Part print with two shaded views. Sizes in mm from the minimum x, y, z corner. A direction names the side the tool comes from. Give positions to 0.01 mm unless a question says otherwise; leave off trailing zeros. Order: outer loops, then holes, each group sorted by start corner. A loop starts at its lowest first (then second) coordinate and runs counter-clockwise, first axis right, second up. Notation, with made-up numbers: M 59.5,55.25 L 90.5,55.25 A29 cw 90.5,78.25 Z; hole C -12,88 d1. An arc over 180 degrees is marked long. Return JSON: item names as keys, results as strings.
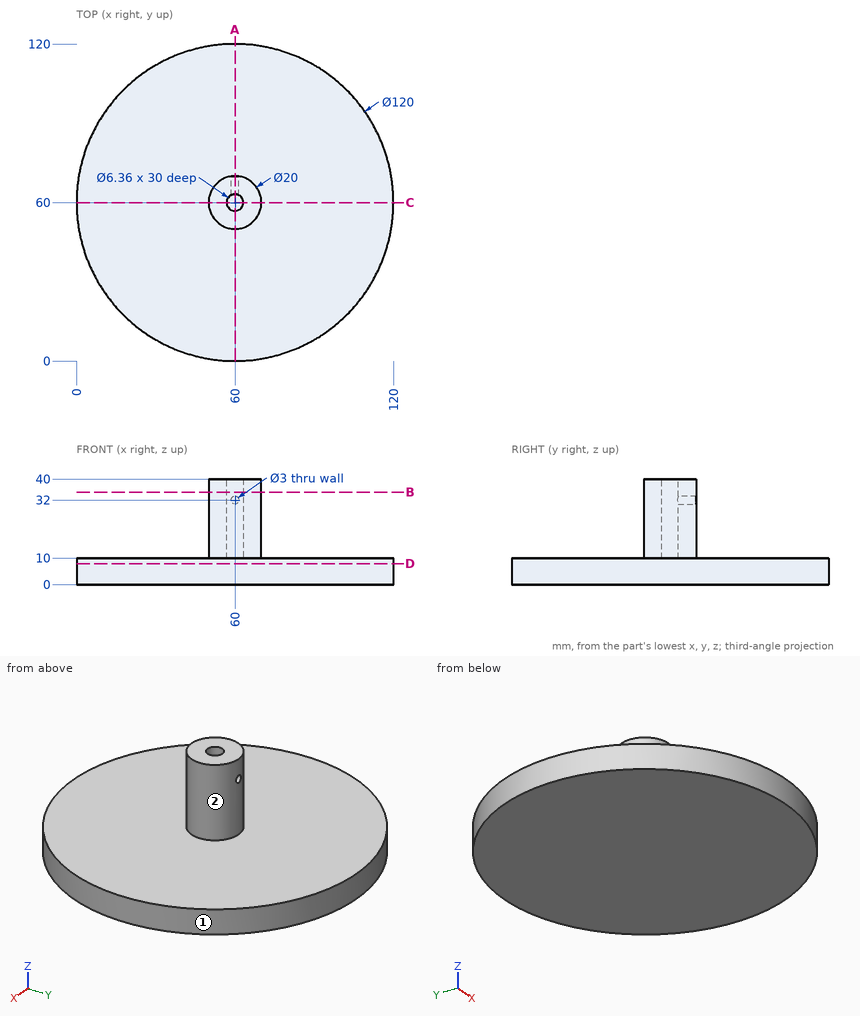
Q1. Band-saw the part on B-B (z = 35). Give the cut face in (x, y).
Established:
{"outline": "C 60,60 d20; hole C 60,60 d6.36"}
Q2. Band-saw the part on C-C (y = 60). Give the cut face in (x, z), then the cut area to 3 significant figures.
Established:
{"outline": "M 0,0 L 120,0 L 120,10 L 70,10 L 70,40 L 63.18,40 L 63.18,10 L 56.82,10 L 56.82,40 L 50,40 L 50,10 L 0,10 Z", "area": "1,610 mm²"}
Q3. Probe line 1 along Y through (x, z) = (60, 17.5); line 2 along Z through (x, y) = (18, 70); line 3 along X through (y, z) = (68, 32). List the from-to ranges inside material, lowest first.
Established:
{"line 1": "y = 50 to 56.82, 63.18 to 70", "line 2": "z = 0 to 10", "line 3": "x = 54 to 58.5, 61.5 to 66"}
Q4. Band-saw the part on A-A (x = 60). Give the cut face in (y, z).
Established:
{"outline": "M 0,0 L 120,0 L 120,10 L 70,10 L 70,30.5 L 63.18,30.5 L 63.18,10 L 56.82,10 L 56.82,40 L 50,40 L 50,10 L 0,10 Z; M 63.18,33.5 L 70,33.5 L 70,40 L 63.18,40 Z"}
Q5. Pin check, flat tips, straight feed: pin 1 (8 mm diameter, centred on x = 97, y = 69.5, fed in from +Z); pin 2 (5 mm diameter, centred on x = 60, z = 32, fed in from -Y); pin 3 (1.5 mm diameter, centred on x = 45.5, z = 4.5, fed in from -Y). Stop position of each tip, or through.
Established:
{"pin 1": "stops at z = 10", "pin 2": "stops at y = 50", "pin 3": "stops at y = 1.6"}
Q6. Band-saw the part on D-D (z = 8). Give the cut face in (x, y), then the cut area to 3 significant figures.
Established:
{"outline": "C 60,60 d120", "area": "11,300 mm²"}
Q7. 3-axis set-ups, long thin cutter, end or side, ignore diameter. For the marked faces 1 and 2: which of +Z, -Z, +X, -X, +Y, -Y reach the whole face in a straight line?
Established:
{"face 1": "+Z, -Z", "face 2": "+Z"}
